Build history of the part. All positions in model axes, mm. Face numbers are marked on the shaded views. A direction names the side the tool comes from. Round coordinates to 2 decimals unless told otherwise and drop trailing zeros. Write each loop counter-clockwise with the first axis right and the second up, starting at its lowest first coordinate (ties: lowest second). Pieces come first, ordered by that corner, then holes.
from build123d import *

# Parameters (mm, degrees)
SKETCH1_W               = 50
SKETCH1_H               = 40
BOSS_EXTRUDE1_DEPTH     = 3.18
SKETCH4_W               = 30
SKETCH4_H               = 4
BOSS_EXTRUDE2_DEPTH     = 36
CUT_EXTRUDE1_DEPTH      = 50.040799341
CUT_EXTRUDE1_DEPTH_BACK = 50.040799341
SKETCH8_W               = 11.6
SKETCH8_H               = 22.1
SKETCH8_R               = 1
SKETCH9_R               = 1.525
CUT_EXTRUDE2_DEPTH      = 49.176757882
FILLET4_R               = 3
SKETCH12_W              = 30
SKETCH12_H              = 2
CUT_EXTRUDE3_DEPTH      = 50.040799341


with BuildPart() as part:
    # Sketch1 → Boss-Extrude1 (new body)
    with BuildSketch(Plane.XY):
        Rectangle(SKETCH1_W, SKETCH1_H)
    extrude(amount=BOSS_EXTRUDE1_DEPTH)

    # Sketch4 → Boss-Extrude2 (add)
    with BuildSketch(Plane(origin=(0, 0, 0), x_dir=(-1, 0, 0), z_dir=(0, 0, -1))):
        Rectangle(SKETCH4_W, SKETCH4_H)
    extrude(amount=BOSS_EXTRUDE2_DEPTH)

    # Sketch8 → Cut-Extrude1 (cut, two sides: drawn at the far end of the back side and taken through both)
    with BuildSketch(Plane(origin=(0, 2, 0), x_dir=(1, 0, 0), z_dir=(0, 1, 0)).offset(-CUT_EXTRUDE1_DEPTH_BACK)):
        with Locations((-5, 19.95)):
            Rectangle(SKETCH8_W, SKETCH8_H)
        with Locations(Location((-5, 6.325, 0), (0, 0, 270))):
            Circle(SKETCH8_R)
    extrude(amount=CUT_EXTRUDE1_DEPTH + CUT_EXTRUDE1_DEPTH_BACK, mode=Mode.SUBTRACT)

    # Sketch9 → Cut-Extrude2 (cut, through all)
    with BuildSketch(Plane(origin=(0, 0, 0), x_dir=(-1, 0, 0), z_dir=(0, 0, -1))):
        with Locations((-18, 12)):
            Circle(SKETCH9_R)
        with Locations((17.0502, 12)):
            Circle(SKETCH9_R)
        with Locations((17.05, -12.889999999)):
            Circle(SKETCH9_R)
        with Locations((-18, -12.889999999)):
            Circle(SKETCH9_R)
    extrude(amount=-CUT_EXTRUDE2_DEPTH, mode=Mode.SUBTRACT)

    # Fillet4
    fillet4_edges = [part.edges().sort_by_distance(p)[0] for p in [
        (0, -2, 0),
    ]]
    fillet(fillet4_edges, radius=FILLET4_R)

    # Sketch12 → Cut-Extrude3 (cut, through all)
    with BuildSketch(Plane.XZ.offset(2)):
        with Locations((0, -35)):
            Rectangle(SKETCH12_W, SKETCH12_H)
    extrude(amount=-CUT_EXTRUDE3_DEPTH, mode=Mode.SUBTRACT)


solid = part.part
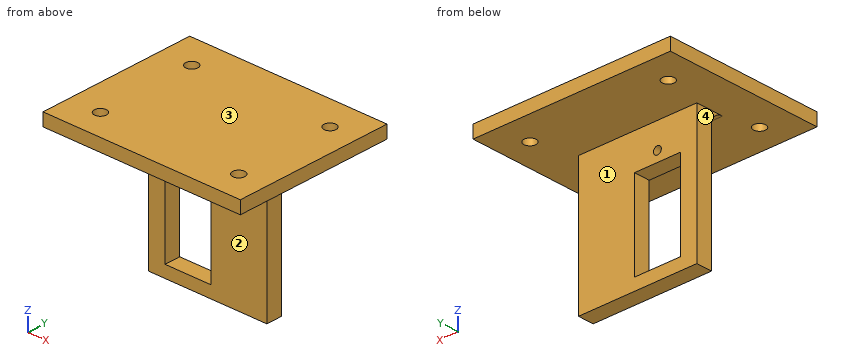
1) Slice it at C-C (y = -1). Write the cut outline in (x, z) (3 decimals), plus the area to 4 significant figures.
Results:
outline: (-25, 0) - (-15, 0) - (-15, -34) - (15, -34) - (15, 0) - (25, 0) - (25, 3.18) - (-25, 3.18) - close; hole (-10.8, -31) - (0.8, -31) - (0.8, -8.9) - (-10.8, -8.9) - close; hole circle Ø2 at (-5, -6.325)
area: 919.5 mm2
2) Slice it at B-B (x = -5). Write the cut outline in (y, z) (3 decimals).
Results:
outline: (-20, 0) - (-5, 0) arc R3 cw to (-2, -3) - (-2, -5.325) - (2, -5.325) - (2, 0) - (20, 0) - (20, 3.18) - (-20, 3.18) - close; (-2, -34) - (2, -34) - (2, -31) - (-2, -31) - close; (-2, -8.9) - (2, -8.9) - (2, -7.325) - (-2, -7.325) - close
3) Slice it at A-A (z = -26). Write the cut outline in (x, y), plus the area to 3 significant figures.
Results:
outline: (-15, -2) - (-10.8, -2) - (-10.8, 2) - (-15, 2) - close; (0.8, -2) - (15, -2) - (15, 2) - (0.8, 2) - close
area: 73.6 mm2
4) Wall check: L1, parallel to Y at x = -17.05, z = 2 (3 decimals); L2, parallel to Y at x = 6, z = -26.5; L3, parallel to Z at x = -4, y = -13.5. Give the ranges that are in metal, low to high.
Results:
L1: y = -20 to -14.415, -11.365 to 10.475, 13.525 to 20
L2: y = -2 to 2
L3: z = 0 to 3.18
5) Pin check, flat tips, straight feed: pin 1 Ø3 at (x, z) = (6, -24.5) entering from +Y; pin 2 Ø4 at (x, y) = (8, -4.5) entering from -Z; pin 3 Ø3 at (y, z) = (0, -15) entering from -X. Stop position of each tip, or through.
Results:
pin 1: stops at y = 2
pin 2: stops at z = -1.34
pin 3: stops at x = -15
6) Slice it at D-D (y = -12.89). Write the cut outline in (x, z) (3 decimals).
Results:
outline: (-25, 0) - (-18.575, 0) - (-18.575, 3.18) - (-25, 3.18) - close; (-15.525, 0) - (16.475, 0) - (16.475, 3.18) - (-15.525, 3.18) - close; (19.525, 0) - (25, 0) - (25, 3.18) - (19.525, 3.18) - close
7) Which spindle directions (+Z, -Z, +X, -X, +Y, -Y) get a long thin tool onto all of the face, cutting with end or side? Do the marked faces 1, 2, 3 and 4. Say none if no direction does.
Results:
face 1: -Z, +X, -X, +Y
face 2: -Z, +X, -X, -Y
face 3: +Z, +X, -X, +Y, -Y
face 4: -Z, -X, +Y, -Y
